```python
from build123d import *

# Parameters (mm, degrees)
BOSS_EXTRUDE1_DEPTH = 3
SKETCH3_R           = 4.5
CUT_EXTRUDE4_DEPTH  = 80.033220863


with BuildPart() as part:
    # Sketch2 → Boss-Extrude1 (new body)
    with BuildSketch(Plane.XY):
        Polygon((0, 64.5), (-8.5, 64.5), (-8.5, 67.5), (-18.5, 67.5), (-18.5, 64.5), (-38, 64.5), (-38, 7.5), (-41, 7.5), (-41, -2.5), (-38, -2.5), (-38, -64.5), (-18.5, -64.5), (-18.5, -67.5), (-8.5, -67.5), (-8.5, -64.5), (0, -64.5), align=None)
    extrude(amount=BOSS_EXTRUDE1_DEPTH)

    # Sketch3 → Cut-Extrude4 (cut, through all)
    with BuildSketch(Plane.XY):
        with Locations((-15, 52.5)):
            Circle(SKETCH3_R)
        with Locations((-15, -52.5)):
            Circle(SKETCH3_R)
    extrude(amount=CUT_EXTRUDE4_DEPTH, mode=Mode.SUBTRACT)


solid = part.part
```
Design review of the part built by this model. Coordinates are the model's own, in mm. A direction names the side the tool comes from. Give positions to 0.01 mm unless a question says otherwise; leave off trailing zeros. Write each loop counter-clockwise with the first axis right and the second up, starting at its lowest first coordinate (ties: lowest second). Pieces come first, ordered by that corner, then holes.
(1) Add section B-B (y = -52.5). Give the boundary of the cut face in (x, z).
Checked values:
outline: (-38, 0) - (-19.5, 0) - (-19.5, 3) - (-38, 3) - close; (-10.5, 0) - (0, 0) - (0, 3) - (-10.5, 3) - close
(2) Add section C-C (z = 0.55). Give the boundary of the cut face in (x, y).
Checked values:
outline: (-41, -2.5) - (-38, -2.5) - (-38, -64.5) - (-18.5, -64.5) - (-18.5, -67.5) - (-8.5, -67.5) - (-8.5, -64.5) - (0, -64.5) - (0, 64.5) - (-8.5, 64.5) - (-8.5, 67.5) - (-18.5, 67.5) - (-18.5, 64.5) - (-38, 64.5) - (-38, 7.5) - (-41, 7.5) - close; hole circle Ø9 at (-15, -52.5); hole circle Ø9 at (-15, 52.5)
(3) Clearance check with flat-ended pins moving along their axes: pin 1 Ø1.5 at (x, z) = (-40, 2) entering from -Y; pin 2 Ø14.5 at (x, y) = (-15, 52.5) entering from +Z; pin 3 Ø1.5 at (y, z) = (66.5, 1.5) entering from -X; pin 4 Ø1.5 at (y, z) = (30, 2) entering from -X. State where each tip first meets the part, or that it passes through.
Checked values:
pin 1: stops at y = -2.5
pin 2: stops at z = 3
pin 3: stops at x = -18.5
pin 4: stops at x = -38
(4) Mouldability with a two-part tool opening along X and no side actions: class faces 1 (the face through (-8.5, -66, 1)), 2 (the face through (-15.98, -56.89, 1.48)), 3 (the face through (-21, 1, 3)) as +X half, -X half, draft (parallel to the pull), parting line (faces both ways), or undercut.
Checked values:
face 1: +X half
face 2: undercut
face 3: draft
(5) Tool access review of faces 4 (the face through (-38, -33, 1)), 5 (the face through (-38, 36, 1)), 6 (the face through (-8.5, 66, 1)): name each direction out of +Z, -Z, +X, -X, +Y, -Y from which nothing blocks a thin tool from reaching the whole face with its end or side.
Checked values:
face 4: +Z, -Z, -X, -Y
face 5: +Z, -Z, -X, +Y
face 6: +Z, -Z, +X, +Y
(6) Add section D-D (x = -24). Give the boundary of the cut face in (y, z).
Checked values:
outline: (-64.5, 0) - (64.5, 0) - (64.5, 3) - (-64.5, 3) - close
(7) Add section A-A (x = -15). Give the boundary of the cut face in (y, z).
Checked values:
outline: (-67.5, 0) - (-57, 0) - (-57, 3) - (-67.5, 3) - close; (-48, 0) - (48, 0) - (48, 3) - (-48, 3) - close; (57, 0) - (67.5, 0) - (67.5, 3) - (57, 3) - close
(8) Wall thickness on line 1 along Y through (x, z) = (-15, 2.05); line 2 along X through (y, z) = (52.5, 2.35); line 3 along Y through (x, z) = (-13, 0.35): over which ranges is each line inside the solid? List them lowest first.
Checked values:
line 1: y = -67.5 to -57, -48 to 48, 57 to 67.5
line 2: x = -38 to -19.5, -10.5 to 0
line 3: y = -67.5 to -56.53, -48.47 to 48.47, 56.53 to 67.5
